Geometry: final body of the model. Coordinates: model frame, mm. Face numbers are marked on the shaded views. A direction names the side the tool comes from. Coordinates: 2 decimals unless noted, no trailing zeros. Order: outer loops, then holes, each group sorted by start corner. A loop starts at its lowest first (then second) coordinate and runs counter-clockwise, first axis right, second up. Notation, with made-up numbers: (-26, 65.5) -> (-13, 65.5) arc R17 ccw to (-13, 77.5) -> close; hole circle Ø8 at (5, -18.5). An arc over 180 degrees is marked (long way). Use CSV: the item, a comma, the result in double quotes. Start each with the question number.
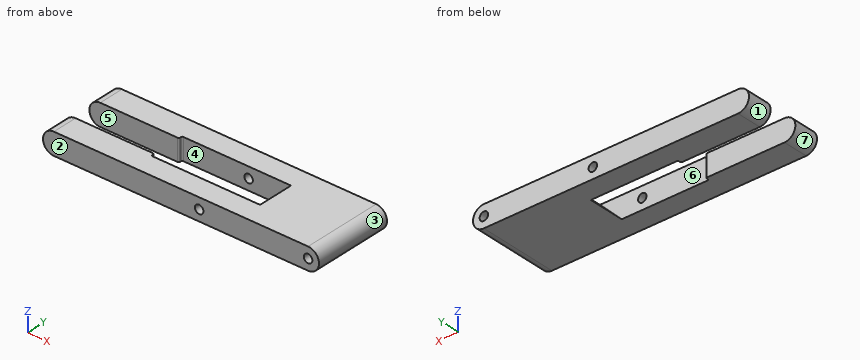
from build123d import *

# Parameters (mm, degrees)
F1_DEPTH    = 16.5
F3_D        = 3.5
F4_W        = 40
F4_H        = 12
F5_DEPTH    = 25
F7_T1_DEPTH = 15
F8_R        = 0.5


# Not quite as in the source:
# - a fillet or chamfer that OpenCascade refuses, or shapes differently, is made with other operations: its cross-section is extruded or revolved along the edge and cut away or added


with BuildPart() as f1:
    # F0 (on Front) → F1 (new body, symmetric)
    with BuildSketch(Plane.XZ):
        with BuildLine():
            ThreePointArc((-52.5, 9), (-57, 4.5), (-52.5, 0))
            Line((-52.5, 0), (52.5, 0))
            ThreePointArc((52.5, 0), (57, 4.5), (52.5, 9))
            Line((52.5, 9), (-52.5, 9))
        make_face()
    extrude(amount=F1_DEPTH, both=True)

    # F3 (through all)
    with Locations(Plane.XZ.offset(16.5)):
        with Locations((7.5, 4.5), (52.5, 4.5)):
            Hole(F3_D / 2)


with BuildPart() as f5:
    # F4 (on Top) → F5 (new body)
    with BuildSketch(Plane.XY):
        Polygon((15, 7.5), (-20, 7.5), (-20, 6), (-20, -6), (-20, -7.5), (15, -7.5), align=None)
        with Locations((-40, 0)):
            Rectangle(F4_W, F4_H)
    extrude(amount=F5_DEPTH)


with BuildPart() as f1_1:
    add(f1.part)

    # F6: cut F5
    add(f5.part, mode=Mode.SUBTRACT)

    # F7: chamfer of 10 on 1 edges, made by hand

    # F7_s2 → F7_t1 (cut)
    with BuildSketch(Plane.XZ.offset(-7.5)):
        with BuildLine():
            Line((25.2828427125, 9.2828427125), (14.7171572875, -1.2828427125))
            Line((14.7171572875, -1.2828427125), (14.5171572875, -1.2828427125))
            ThreePointArc((14.5171572875, -1.2828427125), (14.8, 3.8585786438), (14.8, 9))
            Line((14.8, 9), (15, 9.2))
            ThreePointArc((15, 9.2), (20.1414213562, 9.2), (25.2828427125, 9.4828427125))
            Line((25.2828427125, 9.4828427125), (25.2828427125, 9.2828427125))
        make_face()
    extrude(amount=F7_T1_DEPTH, mode=Mode.SUBTRACT)

    # F8
    f8_edges = [f1_1.edges().sort_by_distance(p)[0] for p in [
        (-20, 7.5, 4.5),
        (-20, 6, 4.5),
        (-20, -7.5, 4.5),
        (-20, -6, 4.5),
    ]]
    fillet(f8_edges, radius=F8_R)


solid = f1_1.part
(1) Section B-B (x = 7.5). Return loops of the section in (y, z), then the cut area to 3 significant figures.
(2) Access query for the marked faces 5, 6 and 7. Directions: +Z, -Z, +X, -X, +Y, -Y. A direction counts if a zero-diameter tool reaches every point of the face in a straight line with its end or side. Return the directions, or none.
(3) Section A-A (z = 4.5). Return loops of the section in (x, y).
(4) First-contact query: pin 1 (1.5 mm diameter, centred on y = 10, z = 5.5, fed in from +X); pin 2 (0.6 mm diameter, centred on y = -6.5, z = 3.5, fed in from +X); pin 3 (1.5 mm diameter, centred on y = 4, z = 4.5, fed in from -X). Flat tips, straight axial feed; report the tip coordinate or a pass-through.
(5) Section C-C (y = 8.5). Return loops of the section in (x, z), then the cut area to 3 significant figures.
(6) Line query: line 1 (X direction, y = 11, z = 4.25); line 2 (Y direction, x = 16, z = 7.5); line 3 (X direction, y = -7, z = 4.75). Output: solid intervals per line, ascending. Write a range as from..to.
(7) Mould query, pull axis X, two halves, no side actions, for the marked faces 1, 2, 3 and 4. Classes: pulls with the +X half, pulls with the -X half, needs draft (parallel to the pull), parting line crosses it, or undercut.
Check sheet entries:
1,outline,"(-16.5, 0) -> (-7.5, 0) -> (-7.5, 2.75) -> (-16.5, 2.75) -> close; (-16.5, 6.25) -> (-7.5, 6.25) -> (-7.5, 9) -> (-16.5, 9) -> close; (7.5, 0) -> (16.5, 0) -> (16.5, 2.75) -> (7.5, 2.75) -> close; (7.5, 6.25) -> (16.5, 6.25) -> (16.5, 9) -> (7.5, 9) -> close"
1,area,"99.0 mm^2"
2,face 5,"+Z, -Z, -X"
2,face 6,"+Z"
2,face 7,"-X, +Y, -Y"
3,outline,"(-57, -16.5) -> (5.75, -16.5) -> (5.75, -7.5) -> (-19.5, -7.5) arc R0.5 cw to (-20, -7) -> (-20, -6.5) arc R0.5 ccw to (-20.5, -6) -> (-57, -6) -> close; (-57, 6) -> (-20.5, 6) arc R0.5 ccw to (-20, 6.5) -> (-20, 7) arc R0.5 cw to (-19.5, 7.5) -> (5.75, 7.5) -> (5.75, 16.5) -> (-57, 16.5) -> close; (9.25, -16.5) -> (50.75, -16.5) -> (50.75, 16.5) -> (9.25, 16.5) -> (9.25, 7.5) -> (20.5, 7.5) -> (20.5, -7.5) -> (9.25, -7.5) -> close; (54.25, -16.5) -> (57, -16.5) -> (57, 16.5) -> (54.25, 16.5) -> close"
4,pin 1,"stops at x = 56.99"
4,pin 2,"stops at x = 56.95"
4,pin 3,"stops at x = 19.75"
5,outline,"(-52.5, 0) -> (52.5, 0) arc R4.5 ccw to (52.5, 9) -> (-52.5, 9) arc R4.5 ccw to start; hole circle Ø3.5 at (7.5, 4.5); hole circle Ø3.5 at (52.5, 4.5)"
5,area,"989 mm^2"
6,line 1,"x = -56.99..5.77, 9.23..50.77, 54.23..56.99"
6,line 2,"y = -16.5..-7.5, 7.5..16.5"
6,line 3,"x = -56.99..-20, 20.75..50.77, 54.23..56.99"
7,face 1,"pulls with the -X half"
7,face 2,"needs draft"
7,face 3,"pulls with the +X half"
7,face 4,"undercut"
